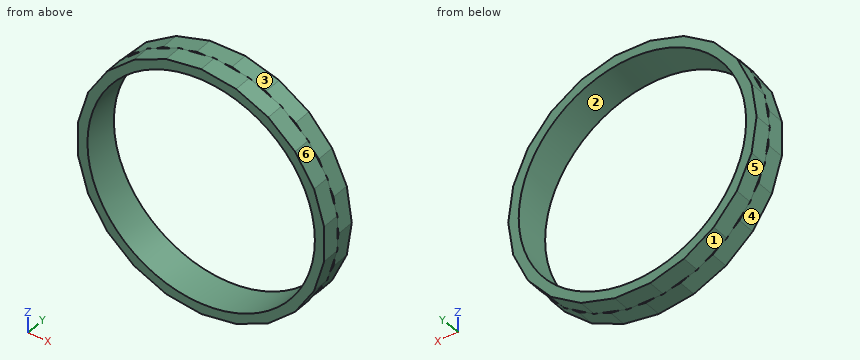
from build123d import *

# Parameters (mm, degrees)
F0_R     = 9.25
F1_DEPTH = 1.5
F2_R     = 9.25
F3_DEPTH = 1.5


with BuildPart() as f1:
    # F0 (on Front) → F1 (new body)
    with BuildSketch(Plane.XZ):
        Polygon((6.615948, 7.635211), (4.196868, 9.189859), (1.437783, 10), (-1.437783, 10), (-4.196868, 9.189859), (-6.615948, 7.635211), (-8.499043, 5.462003), (-9.693597, 2.846297), (-10.102832, 0), (-9.693597, -2.846297), (-8.499043, -5.462003), (-6.615948, -7.635211), (-4.196868, -9.189859), (-1.437783, -10), (1.437783, -10), (4.196868, -9.189859), (6.615948, -7.635211), (8.499043, -5.462003), (9.693597, -2.846297), (10.102832, 0), (9.693597, 2.846297), (8.499043, 5.462003), align=None)
        Circle(F0_R, mode=Mode.SUBTRACT)
    extrude(amount=F1_DEPTH)

    # F2 (on face) → F3 (join)
    with BuildSketch(Plane.XZ.offset(1.5)):
        Polygon((5.462003, 8.499043), (2.846297, 9.693597), (0, 10.102832), (-2.846297, 9.693597), (-5.462003, 8.499043), (-7.635211, 6.615948), (-9.189859, 4.196868), (-10, 1.437783), (-10, -1.437783), (-9.189859, -4.196868), (-7.635211, -6.615948), (-5.462003, -8.499043), (-2.846297, -9.693597), (0, -10.102832), (2.846297, -9.693597), (5.462003, -8.499043), (7.635211, -6.615948), (9.189859, -4.196868), (10, -1.437783), (10, 1.437783), (9.189859, 4.196868), (7.635211, 6.615948), align=None)
        Circle(F2_R, mode=Mode.SUBTRACT)
    extrude(amount=F3_DEPTH)


solid = f1.part
Model file for the job. Use its own axes, mm. Face numbers are marked on the shaded views. A direction names the side the tool comes from. Give positions to 0.01 mm unless a question says otherwise; leave off trailing zeros. Write each loop counter-clockwise with the first axis right and the second up, starting at its lowest first coordinate (ties: lowest second). Pieces come first, ordered by that corner, then holes. Notation, with made-up numbers: (32, 23) - (69, 23) arc R16 ccw to (69, 43) - close; hole circle Ø6 at (-12.75, 78.25). An arc over 180 degrees is marked (long way). Answer as CSV lines item,"result".
1. Band-saw the part on B-B (z = -2.5). Write the cut outline in (x, y).
Responses:
outline,"(-9.74, -1.5) - (-9.69, -1.5) - (-9.69, -3) - (-8.91, -3) - (-8.91, 0) - (-9.74, 0) - close; (8.91, -3) - (9.69, -3) - (9.69, -1.5) - (9.74, -1.5) - (9.74, 0) - (8.91, 0) - close"
2. Drill centre lines: L1, parallel to Z at x = 0, y = -2.3; L2, parallel to Z at x = 0, y = -1.1; L3, parallel to X at y = -2.55, z = -2.75. Where is each one in solid material? Low to high. Write a range as [from, to].
Responses:
L1,"z = [-10.1, -9.25], [9.25, 10.1]"
L2,"z = [-10, -9.25], [9.25, 10]"
L3,"x = [-9.61, -8.83], [8.83, 9.61]"
3. Pin check, flat tips, straight feed: pin 1 (1 mm diameter, centred on y = -2, z = -2, fed in from +X); pin 2 (12 mm diameter, centred on x = 0, z = 5.5, fed in from +Y). Stop position of each tip, or through.
Responses:
pin 1,"stops at x = 9.98"
pin 2,"stops at y = 0"
4. Band-saw the part on A-A (y = -0.35). Write the cut outline in (x, z).
Responses:
outline,"(-10.1, 0) - (-9.69, -2.85) - (-8.5, -5.46) - (-6.62, -7.64) - (-4.2, -9.19) - (-1.44, -10) - (1.44, -10) - (4.2, -9.19) - (6.62, -7.64) - (8.5, -5.46) - (9.69, -2.85) - (10.1, 0) - (9.69, 2.85) - (8.5, 5.46) - (6.62, 7.64) - (4.2, 9.19) - (1.44, 10) - (-1.44, 10) - (-4.2, 9.19) - (-6.62, 7.64) - (-8.5, 5.46) - (-9.69, 2.85) - close; hole circle Ø18.5 at (0, 0)"
5. Two-plate mould, pull along Z, no slides. Class the marked faces 1, 2 and 3: +Z half, -Z half, draft (parallel to the pull), parting line (faces both ways), or undercut.
Responses:
face 1,"-Z half"
face 2,"undercut"
face 3,"+Z half"
6. 3-axis set-ups, long thin cutter, end or side, ignore diameter. For the marked faces 4, 5 and 6: which of +Z, -Z, +X, -X, +Y, -Y reach the whole face in a straight line?
Responses:
face 4,"-Z, -X, -Y"
face 5,"-Z, -X, +Y"
face 6,"+Z, +X, -Y"
